Source: CAD feature listing. Evaluate the final solid. Frame: model axes, mm. A direction names the side the tool comes from. Coordinates: 2 decimals unless noted, no trailing zeros. Loops run counter-clockwise (first coordinate to the right, second up) from the corner with the lowest first, then second, coordinate; pieces in that order, holes last.
```python
from build123d import *

# Parameters (mm, degrees)
ESQUISSE1_R             = 6.35
ESQUISSE1_R_2           = 9.5
BOSS_EXTRU_1_DEPTH      = 28.5
ENL_V_START             = -6
ENL_V_MAT_EXTRU_1_DEPTH = 6
ENL_V_MAT_EXTRU_2_DEPTH = 6
ESQUISSE4_W             = 38
ESQUISSE4_H             = 14.5
ENL_V_MAT_EXTRU_3_DEPTH = 124.584469767


with BuildPart() as part:
    # Esquisse1 → Boss.-Extru.1 (new body)
    with BuildSketch(Plane.XY):
        with BuildLine():
            Line((-86.633280406, -6.99307262), (-81.912918385, -55.104590809))
            ThreePointArc((-81.912918385, -55.104590809), (-74.795399572, -69.254576275), (-60.018047616, -74.956420883))
            Line((-60.018047616, -74.956420883), (-1.018047616, -74.956420883))
            Line((-1.018047616, -74.956420883), (-1.018047616, -59.456420883))
            Line((-1.018047616, -59.456420883), (-23.018047616, -59.456420883))
            ThreePointArc((-23.018047616, -59.456420883), (-29.518047616, -52.956420883), (-23.018047616, -46.456420883))
            Line((-23.018047616, -46.456420883), (-1.018047616, -46.456420883))
            Line((-1.018047616, -46.456420883), (-1.018047616, -38.956420883))
            ThreePointArc((-1.018047616, -38.956420883), (-35.318453229, -28.420111536), (-59.263146108, -1.695902984))
            ThreePointArc((-59.263146108, -1.695902984), (-75.360354059, 8.118888343), (-86.633280406, -6.99307262))
        make_face()
        with Locations(Location((-72.700180587, -5.626055331, 0), (0, 0, 180))):
            Circle(ESQUISSE1_R, mode=Mode.SUBTRACT)
        with Locations(Location((-60.018047616, -52.956420883, 0), (0, 0, 180))):
            Circle(ESQUISSE1_R_2, mode=Mode.SUBTRACT)
    extrude(amount=BOSS_EXTRU_1_DEPTH)

    # Esquisse2 → Enlèv. mat.-Extru.1 (cut)
    with BuildSketch(Plane.XY.offset(28.5).offset(ENL_V_START)):
        with BuildLine():
            Line((-50.888781824, -14.626055395), (-55.966980296, -14.626055395))
            ThreePointArc((-55.966980296, -14.626055395), (-69.422632675, -24.341227799), (-85.379019392, -19.776922952))
            Line((-85.379019392, -19.776922952), (-86.633280406, -6.99307262))
            ThreePointArc((-86.633280406, -6.99307262), (-75.360354059, 8.118888343), (-59.263146108, -1.695902984))
            ThreePointArc((-59.263146108, -1.695902984), (-55.448825079, -8.402467045), (-50.888781824, -14.626055395))
        make_face()
    extrude(amount=ENL_V_MAT_EXTRU_1_DEPTH, mode=Mode.SUBTRACT)

    # Esquisse3 → Enlèv. mat.-Extru.2 (cut)
    with BuildSketch(Plane(origin=(0, 0, 0), x_dir=(-1, 0, 0), z_dir=(0, 0, -1))):
        with BuildLine():
            Line((85.379019392, -19.776922952), (86.633280406, -6.99307262))
            ThreePointArc((86.633280406, -6.99307262), (75.360354059, 8.118888343), (59.263146108, -1.695902984))
            ThreePointArc((59.263146108, -1.695902984), (55.448825079, -8.402467045), (50.888781824, -14.626055395))
            Line((50.888781824, -14.626055395), (55.966980296, -14.626055395))
            ThreePointArc((55.966980296, -14.626055395), (69.422632675, -24.341227799), (85.379019392, -19.776922952))
        make_face()
    extrude(amount=-ENL_V_MAT_EXTRU_2_DEPTH, mode=Mode.SUBTRACT)

    # Esquisse4 → Enlèv. mat.-Extru.3 (cut, through all)
    with BuildSketch(Plane.XZ.offset(74.956420883)):
        with Locations((-20.018047616, 14.25)):
            Rectangle(ESQUISSE4_W, ESQUISSE4_H)
    extrude(amount=-ENL_V_MAT_EXTRU_3_DEPTH, mode=Mode.SUBTRACT)


solid = part.part
```
Q1. Section query A-A on x = -54.5. Return the cut outline in (y, z).
Q2. Draft query along X for faces 4 (the flat face through (-44, -51, 28.5)), 5 (the flat face through (-1.018, -43, 3)), 6 (the flat face through (-84.306, -30.712, 14.05)), 7 (the cylindrical face through (-78.76, -7.53, 14.13)). Return one class per face: released by +X, released by -X, zero draft, split by the parting line, or undercut.
Q3. Section query D-D on z = 17.25. Return the cut outline in (x, y).
Q4. First-contact query: pin 1 Ø2 at (x, z) = (-16.5, 24.5) entering from +Y; pin 2 Ø1.5 at (y, z) = (-19, 22) entering from +X; pin 3 Ø4 at (x, z) = (-52.5, 2.5) entering from +Y. Flat tips, straight axial feed; report the tip coordinate or a pass-through.
Q5. Reachability of faces 1 (the flat face through (-53, -14.626, 25)), 2 (the flat face through (-53, -14.626, 3)), 3 (the cylindrical face through (-69.2, -24.3, 3)) from +Z, -Z, +X, -X, +Y, -Y: full face, straight path, thin tool, end or side. Return the list, or none.
Q6. Section query B-B on z = 23.5. Return the cut outline in (x, y).
Q7. Material intervals for line 1 along Z through (x, y) = (-37.5, -43); line 2 along Z through (x, y) = (-52, -14); line 3 along Y through (x, z) = (-25, 6.25), sorted ascending.
Q8. Section query C-C on y = -67. Return the cut outline in (x, z).
Resolved:
1. outline: (-74.96, 0) - (-60.69, 0) - (-60.69, 28.5) - (-74.96, 28.5) - close; (-45.22, 0) - (-14.63, 0) - (-14.63, 6) - (-9.83, 6) - (-9.83, 22.5) - (-14.63, 22.5) - (-14.63, 28.5) - (-45.22, 28.5) - close
2. face 4: zero draft
2. face 5: released by +X
2. face 6: released by -X
2. face 7: undercut
3. outline: (-86.63, -6.99) - (-81.91, -55.1) arc R22 ccw to (-60.02, -74.96) - (-39.02, -74.96) - (-39.02, -25.87) arc R67 cw to (-59.26, -1.7) arc R14 ccw to start; hole circle Ø12.7 at (-72.7, -5.63); hole circle Ø19 at (-60.02, -52.96)
4. pin 1: stops at y = -36.44
4. pin 2: stops at x = -46.19
4. pin 3: stops at y = -14.63
5. face 1: +Z, +X, -X, +Y
5. face 2: -Z, +X, -X, +Y
5. face 3: -Z, +Y
6. outline: (-85.38, -19.78) - (-81.91, -55.1) arc R22 ccw to (-60.02, -74.96) - (-1.02, -74.96) - (-1.02, -59.46) - (-23.02, -59.46) arc R6.5 cw to (-23.02, -46.46) - (-1.02, -46.46) - (-1.02, -38.96) arc R67 cw to (-50.89, -14.63) - (-55.97, -14.63) arc R19 cw to start; hole circle Ø19 at (-60.02, -52.96)
7. line 1: z = 0 to 7, 21.5 to 28.5
7. line 2: z = 6 to 22.5
7. line 3: y = -74.96 to -59.15, -46.77 to -33.82
8. outline: (-76.95, 0) - (-1.02, 0) - (-1.02, 7) - (-39.02, 7) - (-39.02, 21.5) - (-1.02, 21.5) - (-1.02, 28.5) - (-76.95, 28.5) - close
